Here's the drawing with two shaded views (mm, measured from the low corner). I have some questions. Give positions to 0.01 mm unless a question says otherwise; leave off trailing zeros. Loops run counter-clockwise (first coordinate to the right, second up) from the corner with the lowest first, then second, coordinate; pieces in that order, holes last. Notation, with made-up numbers: (36, -19) -> (77, -19) arc R29 ccw to (77, 14) -> close; hole circle Ø7 at (77, 20). An arc over 180 degrees is marked (long way). Put each result on its own line as item: value.
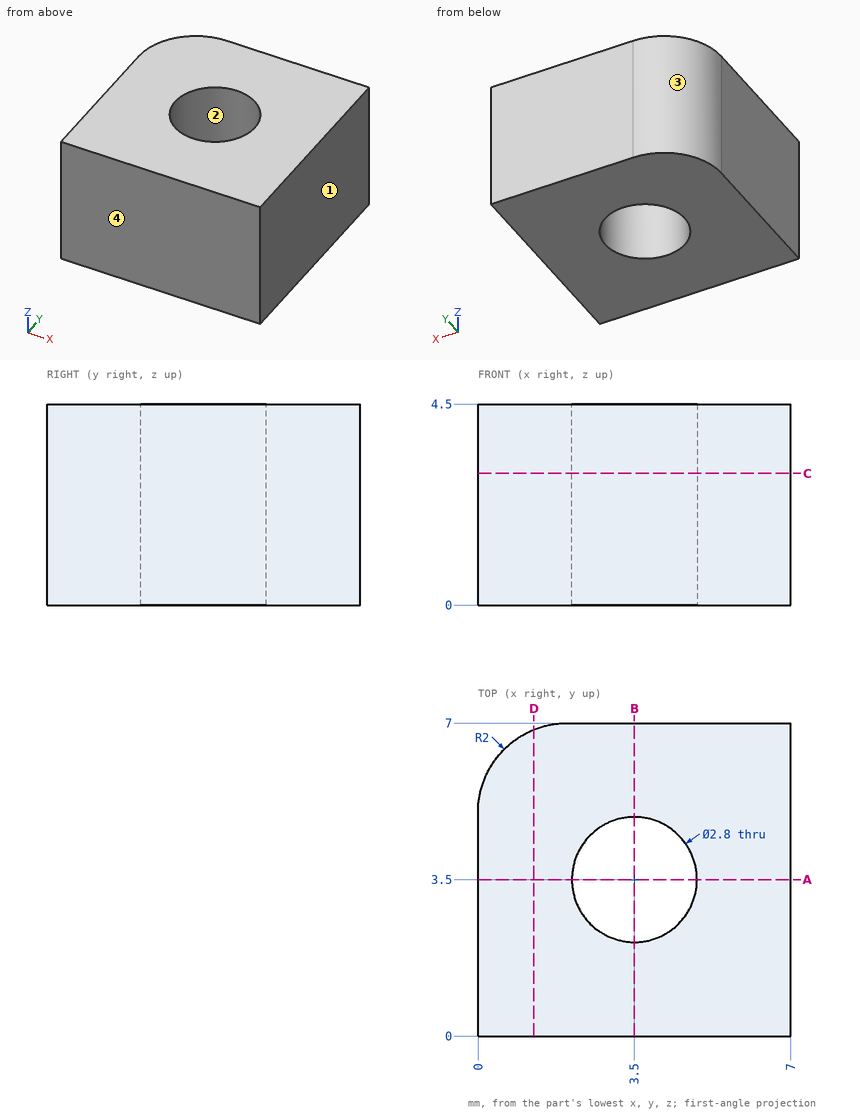
1. If we section it at D-D (x = 1.25): List the corners of the cut face in (y, z) for me.
Recorded:
outline: (0, 0) -> (6.85, 0) -> (6.85, 4.5) -> (0, 4.5) -> close
2. I'm going to push a flat-ended pin straight in: pin 1 (2.5 mm diameter, centred on x = 3.5, y = 3.5, fed in from -Z). Where does the tip first touch, or does it pass through?
Recorded:
pin 1: passes through
3. Thinking about a two-plate mould opening in X: for the marked faces 1, 2, 3 and 4, which applies, pulls with the +X half, pulls with the -X half, needs draft (parallel to the pull), parting line crosses it, or undercut?
Recorded:
face 1: pulls with the +X half
face 2: undercut
face 3: pulls with the -X half
face 4: needs draft
4. If we section it at C-C (z = 2.95): List the corners of the cut face in (x, y) for me.
Recorded:
outline: (0, 0) -> (7, 0) -> (7, 7) -> (2, 7) arc R2 ccw to (0, 5) -> close; hole circle Ø2.8 at (3.5, 3.5)
5. I need wall thicknesses on line 1 (Y direction, x = 3.5, z = 2.8); line 2 (X direction, y = 4.5, z = 0.9); line 3 (Y direction, x = 1, z = 0.6). Which ranges of each line are inside material? Lowest first, please.
Recorded:
line 1: y = 0 to 2.1, 4.9 to 7
line 2: x = 0 to 2.52, 4.48 to 7
line 3: y = 0 to 6.73
6. If we section it at A-A (y = 3.5): List the corners of the cut face in (x, z) for me, then the cut area to 3 significant figures.
Recorded:
outline: (0, 0) -> (2.1, 0) -> (2.1, 4.5) -> (0, 4.5) -> close; (4.9, 0) -> (7, 0) -> (7, 4.5) -> (4.9, 4.5) -> close
area: 18.9 mm^2
